from build123d import *

# Parameters (mm, degrees)
SKETCH1_R             = 150
SKETCH1_R_2           = 11
BOSS_EXTRUDE1_DEPTH   = 20
F_6_0MM_DOWEL_HOLE1_D = 6
F_8_0MM_DOWEL_HOLE1_D = 8
CIRPATTERN2_COUNT     = 4
CUT_EXTRUDE2_DEPTH    = 1
CIRPATTERN3_COUNT     = 8
SKETCH2_R             = 12.5
CUT_EXTRUDE4_DEPTH    = 214.072757527
CIRPATTERN4_COUNT     = 4


with BuildPart() as part:
    # Sketch1 → Boss-Extrude1 (new body)
    with BuildSketch(Plane.XY):
        Circle(SKETCH1_R)
        Circle(SKETCH1_R_2, mode=Mode.SUBTRACT)
    extrude(amount=BOSS_EXTRUDE1_DEPTH)

    # Ø6.0mm Dowel Hole1 (through all)
    with Locations(Plane(origin=(0, 0, 0), x_dir=(-1, 0, 0), z_dir=(0, 0, -1))):
        with Locations((-15.705952053, -6.50561835)):
            f_6_0mm_dowel_hole1 = Hole(F_6_0MM_DOWEL_HOLE1_D / 2)

    # Ø8.0mm Dowel Hole1 (through all)
    with Locations(Plane(origin=(0, 0, 0), x_dir=(-1, 0, 0), z_dir=(0, 0, -1))):
        with Locations((-32.335783638, -13.393920133)):
            f_8_0mm_dowel_hole1 = Hole(F_8_0MM_DOWEL_HOLE1_D / 2)

    # CirPattern2: Ø6.0mm Dowel Hole1, Ø8.0mm Dowel Hole1 ×4 about axis
    cirpattern2_axis = Axis((0, 0, 0), (0, 0, 1))
    add([f_6_0mm_dowel_hole1.rotate(cirpattern2_axis, i * 360 / CIRPATTERN2_COUNT) for i in range(1, CIRPATTERN2_COUNT)], mode=Mode.SUBTRACT)
    add([f_8_0mm_dowel_hole1.rotate(cirpattern2_axis, i * 360 / CIRPATTERN2_COUNT) for i in range(1, CIRPATTERN2_COUNT)], mode=Mode.SUBTRACT)

    # Sketch9 → Cut-Extrude2 (cut)
    with BuildSketch(Plane.XY.offset(20)):
        Polygon((-42.426406871, 105.926406871), (0.707106781, 62.792893219), (43.840620434, 105.926406871), (0.707106781, 149.059920524), align=None)
    cut_extrude2 = extrude(amount=-CUT_EXTRUDE2_DEPTH, mode=Mode.SUBTRACT)

    # CirPattern3: Cut-Extrude2 ×8 about axis
    cirpattern3_axis = Axis((0, 0, 0), (0, 0, 1))
    for i in range(1, CIRPATTERN3_COUNT):
        add(cut_extrude2.rotate(cirpattern3_axis, i * 360 / CIRPATTERN3_COUNT), mode=Mode.SUBTRACT)

    # Sketch2 → Cut-Extrude4 (cut, through all)
    with BuildSketch(Plane.XY):
        with Locations((43.422338028, 17.986121321)):
            Circle(SKETCH2_R)
    cut_extrude4 = extrude(amount=CUT_EXTRUDE4_DEPTH, mode=Mode.SUBTRACT)

    # CirPattern4: Cut-Extrude4 ×4 about axis
    cirpattern4_axis = Axis((0, 0, 0), (0, 0, 1))
    for i in range(1, CIRPATTERN4_COUNT):
        add(cut_extrude4.rotate(cirpattern4_axis, i * 360 / CIRPATTERN4_COUNT), mode=Mode.SUBTRACT)


solid = part.part
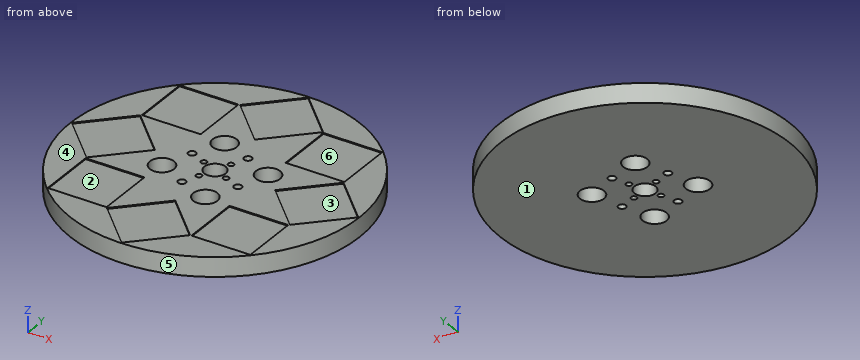
The listing builds one solid part. Answer for the finished solid, in the listing's coordinates (mm). Face numbers are marked on the shaded views. A direction names the side the tool comes from. Give positions to 0.01 mm unless a question says otherwise; leave off trailing zeros. Loops run counter-clockwise (first coordinate to the right, second up) from the corner with the lowest first, then second, coordinate; pieces in that order, holes last. Notation, with made-up numbers: (-36.5, 4) - (17.5, 4) arc R17 cw to (17.5, 33) - close; hole circle Ø11 at (58, -1.5). An arc over 180 degrees is marked (long way). Use one line per item in the form item = value.
1. Given pin 1 Ø10 at (x, y) = (-80.5, -107.5) entering from -Z; pin 2 Ø0.5 at (y, z) = (61, 19.5) entering from -X; pin 3 Ø0.5 at (y, z) = (-82, 19.5) entering from -X; pin 4 Ø10 at (x, z) = (-72.5, 6.5) entering from -Y, each flat-ended and moving along its own axis, determine where each tip first touches the part or whether it passes through.
Calculated:
pin_1 = 0
pin_2 = -137.15
pin_3 = -125.77
pin_4 = -133.95
2. Section D-D on y = 125 is taken. Give the vertices of the cut face in (x, z), then the cut area to 3 significant figures.
Calculated:
outline = (-82.92, 0) - (82.92, 0) - (82.92, 20) - (24.77, 20) - (24.77, 19) - (-23.35, 19) - (-23.35, 20) - (-82.92, 20) - close
area = 3,270 mm^2
3. The mould has two halves that part along Y. Classify the marked faces 3, 4, 5 and 6: pulls with the +Y half, pulls with the -Y half, needs draft (parallel to the pull), parting line crosses it, or undercut.
Calculated:
face_3 = undercut
face_4 = needs draft
face_5 = parting line crosses it
face_6 = undercut
4. Which of the six approach directions +Z, -Z, +X, -X, +Y, -Y give full straight-line access (tool end or side, diameter ignored) to the marked faces 1 and 2?
Calculated:
face_1 = -Z, +X, -X, +Y, -Y
face_2 = +Z
5. Section C-C on x = 124.5 is taken. Give the vertices of the cut face in (y, z), then the cut area to 3 significant figures.
Calculated:
outline = (-83.66, 0) - (83.66, 0) - (83.66, 20) - (23.85, 20) - (23.85, 19) - (-25.27, 19) - (-25.27, 20) - (-83.66, 20) - close
area = 3,300 mm^2
6. Find the intervals of material crossed by line 1 along Y through (x, z) = (-7.5, 10.5); line 2 along Y through (x, z) = (-34.5, 10); line 3 along Y through (x, z) = (0, 10), in increasing order. Write a range as [from, to].
Calculated:
line_1 = [-149.81, -18.54], [-12.88, -8.05], [8.05, 36.62], [50.23, 149.81]
line_2 = [-145.98, -26.74], [-9.23, 10.03], [16.76, 145.98]
line_3 = [-150, -11], [11, 150]
7. Section B-B on y = -87.5 is taken. Give the vertices of the cut face in (x, z), then the cut area to 3 significant figures.
Calculated:
outline = (-121.83, 0) - (121.83, 0) - (121.83, 20) - (104.9, 20) - (104.9, 19) - (43.9, 19) - (43.9, 20) - (24, 20) - (24, 19) - (-25.41, 19) - (-25.41, 20) - (-44.9, 20) - (-44.9, 19) - (-105.9, 19) - (-105.9, 20) - (-121.83, 20) - close
area = 4,700 mm^2
8. Section A-A on z = 15 is taken. Count the separate pieces of the cut face and the enclosed holes in it, then the cut area to 3 significant figures.
Calculated:
separate_pieces = 1
enclosed_holes = 13
area = 68,000 mm^2
